Answer from the drawing. Dimensions are ordinates in mm from the lowest x, y and z of the part. A direction names the side the tool comes from. Coordinates: 2 decimals unless noted, no trailing zeros. Loops run counter-clockwise (first coordinate to the right, second up) from the corner with the lowest first, then second, coordinate; pieces in that order, holes last. Notation, with made-up numbers: M 31.5,-38 L 57.5,-38 A36 cw 57.5,-3 Z; hole C 47,0.5 d2. An arc over 180 degrees is marked long. Put each result on its own line as item: value.
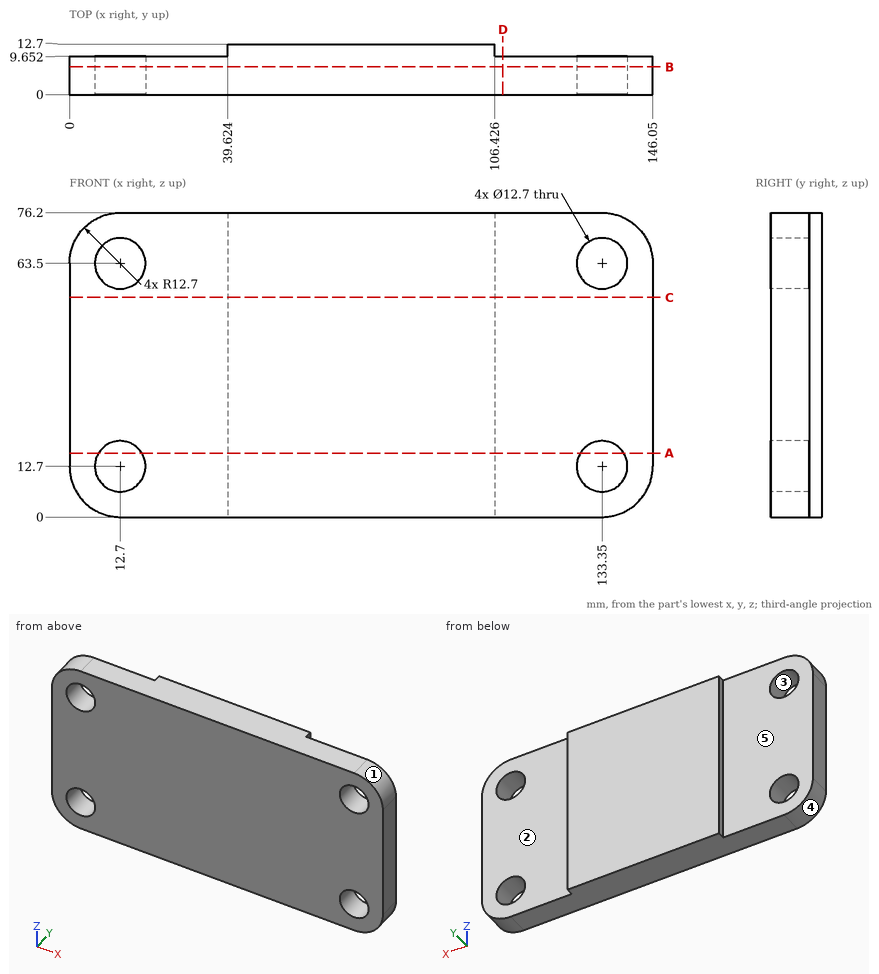
1) Find section B-B, the plane y = 7. Write down the section's boundary in (x, z).
Answer list:
outline: M 0,12.7 A12.7 ccw 12.7,0 L 133.35,0 A12.7 ccw 146.05,12.7 L 146.05,63.5 A12.7 ccw 133.35,76.2 L 12.7,76.2 A12.7 ccw 0,63.5 Z; hole C 12.7,12.7 d12.7; hole C 12.7,63.5 d12.7; hole C 133.35,12.7 d12.7; hole C 133.35,63.5 d12.7
2) Determine the mould class of the marked faces 3, 4 and 5 for opening direction X: released by +X, released by -X, zero draft, split by the parting line, or undercut.
Answer list:
face 3: undercut
face 4: released by -X
face 5: zero draft
3) Given pin 1 Ø16.5 at (x, z) = (133.35, 12.7) entering from +Y; pin 2 Ø1.5 at (y, z) = (10.5, 29) entering from +X; pin 3 Ø7.5 at (x, z) = (12.7, 12.7) entering from -Y, each flat-ended and moving along its own axis, determine where each tip first touches the part or whether it passes through.
Answer list:
pin 1: stops at y = 9.65
pin 2: stops at x = 106.43
pin 3: passes through
4) Straight lines are drawn through the part: line 1 (Z direction, x = 12.7, y = 5.75); line 2 (Z direction, x = 18, y = 8); line 3 (Y direction, x = 122.5, z = 28.5). For each, find the intervals that lie inside material, in ascending order. Write a range as [from, to].
Answer list:
line 1: z = [0, 6.35], [19.05, 57.15], [69.85, 76.2]
line 2: z = [0, 9.2], [16.2, 60], [67, 76.2]
line 3: y = [0, 9.65]
5) Find section D-D, the plane x = 108.5. Write down the section's boundary in (y, z), plus the area to 3 significant figures.
Answer list:
outline: M 0,0 L 9.65,0 L 9.65,76.2 L 0,76.2 Z
area: 735 mm^2
6) Find section C-C, the plane z = 55. Write down the section's boundary in (x, y).
Answer list:
outline: M 0,0 L 146.05,0 L 146.05,9.65 L 106.43,9.65 L 106.43,12.7 L 39.62,12.7 L 39.62,9.65 L 0,9.65 Z
7) Find section A-A, the plane z = 16. Write down the section's boundary in (x, y), plus the area to 3 significant figures.
Answer list:
outline: M 0,0 L 7.27,0 L 7.27,9.65 L 0,9.65 Z; M 18.13,0 L 127.92,0 L 127.92,9.65 L 106.43,9.65 L 106.43,12.7 L 39.62,12.7 L 39.62,9.65 L 18.13,9.65 Z; M 138.78,0 L 146.05,0 L 146.05,9.65 L 138.78,9.65 Z
area: 1,400 mm^2
8) Which of the six approach directions +Z, -Z, +X, -X, +Y, -Y give full straight-line access (tool end or side, diameter ignored) to the marked faces 1 and 2?
Answer list:
face 1: +Z, +X, +Y, -Y
face 2: +Z, -Z, +X, +Y
